from build123d import *

# Parameters (mm, degrees)
ESQUISSE1_W             = 54
ESQUISSE1_H             = 18
ESQUISSE1_R             = 3
BOSS_EXTRU_1_DEPTH      = 59
ESQUISSE2_W             = 89.885876072
ESQUISSE2_H             = 74.564815434
ENL_V_MAT_EXTRU_1_DEPTH = 13
D_GAGEMENT_M101_D       = 11


with BuildPart() as part:
    # Esquisse1 → Boss.-Extru.1 (new body)
    with BuildSketch(Plane.XY):
        Rectangle(ESQUISSE1_W, ESQUISSE1_H)
        with Locations((-19, 2)):
            Circle(ESQUISSE1_R, mode=Mode.SUBTRACT)
        with Locations((21, 2)):
            Circle(ESQUISSE1_R, mode=Mode.SUBTRACT)
    extrude(amount=BOSS_EXTRU_1_DEPTH)

    # Esquisse2 → Enlèv. mat.-Extru.1 (cut)
    with BuildSketch(Plane(origin=(0, 9, 0), x_dir=(1, 0, 0), z_dir=(0, 1, 0))):
        with Locations((-2.437014962, -42.282407717)):
            Rectangle(ESQUISSE2_W, ESQUISSE2_H)
    extrude(amount=-ENL_V_MAT_EXTRU_1_DEPTH, mode=Mode.SUBTRACT)

    # Dégagement M101 (through all)
    with Locations(Plane(origin=(0, -4, 0), x_dir=(1, 0, 0), z_dir=(0, 1, 0))):
        with Locations((9.500000001, -45.5022105)):
            Hole(D_GAGEMENT_M101_D / 2)


solid = part.part
Could you check a few things on this model? Use its own coordinates, in mm. A direction names the side the tool comes from. Coordinates: 2 decimals unless noted, no trailing zeros. Loops run counter-clockwise (first coordinate to the right, second up) from the corner with the lowest first, then second, coordinate; pieces in that order, holes last.
1. For P1, Ø7, axis at x = -19, y = 2, coming from the +Z side; P2, Ø2, axis at x = -17, z = 31, coming from the +Y side, each with a flat end and sliding along its axis, tell me the tip position at first contact or that it passes through.
2. Imagine slicing it at A-A (x = 21). Please give me the cut outline in (y, z).
3. We'd pull the mould along X, two halves only. Please class faces 3 (the face through (27, -6, 23)), 4 (the face through (0, 0, 0)), 5 (the face through (-22, 2, 2)): released by +X, released by -X, zero draft, split by the parting line, or undercut.
4. Imagine slicing it at C-C (z = 48). Please give me the cut outline in (x, y), and give its area (3 significant figures).
5. Imagine slicing it at B-B (y = 2). Please give me the cut outline in (x, z).
6. For faces 1 (the face through (18, 2, 2)), 2 (the face through (0, -4, 32)), which set-ups out of +Z, -Z, +X, -X, +Y, -Y let a thin tool reach every point of the face, with its end or its side?
7. Imagine slicing it at D-D (x = 9.5). Please give me the cut outline in (y, z).
8. I need wall thicknesses on L1, parallel to X at y = 2, z = 1.6; L2, parallel to Y at x = 21, z = 3.25; L3, parallel to Z at x = 9.5, y = -7.85. Which ranges of each line are inside material? Lowest first, please.
Computed values:
1. P1: stops at z = 5
1. P2: stops at y = -4
2. outline: (-9, 0) - (-1, 0) - (-1, 5) - (-4, 5) - (-4, 59) - (-9, 59) - close; (5, 0) - (9, 0) - (9, 5) - (5, 5) - close
3. face 3: released by +X
3. face 4: zero draft
3. face 5: undercut
4. outline: (-27, -9) - (4.6, -9) - (4.6, -4) - (-27, -4) - close; (14.4, -9) - (27, -9) - (27, -4) - (14.4, -4) - close
4. area: 221 mm2
5. outline: (-27, 0) - (-22, 0) - (-22, 5) - (-27, 5) - close; (-16, 0) - (18, 0) - (18, 5) - (-16, 5) - close; (24, 0) - (27, 0) - (27, 5) - (24, 5) - close
6. face 1: +Z, -Z
6. face 2: +Z, +X, -X, +Y
7. outline: (-9, 0) - (9, 0) - (9, 5) - (-4, 5) - (-4, 40) - (-9, 40) - close; (-9, 51) - (-4, 51) - (-4, 59) - (-9, 59) - close
8. L1: x = -27 to -22, -16 to 18, 24 to 27
8. L2: y = -9 to -1, 5 to 9
8. L3: z = 0 to 40, 51 to 59
